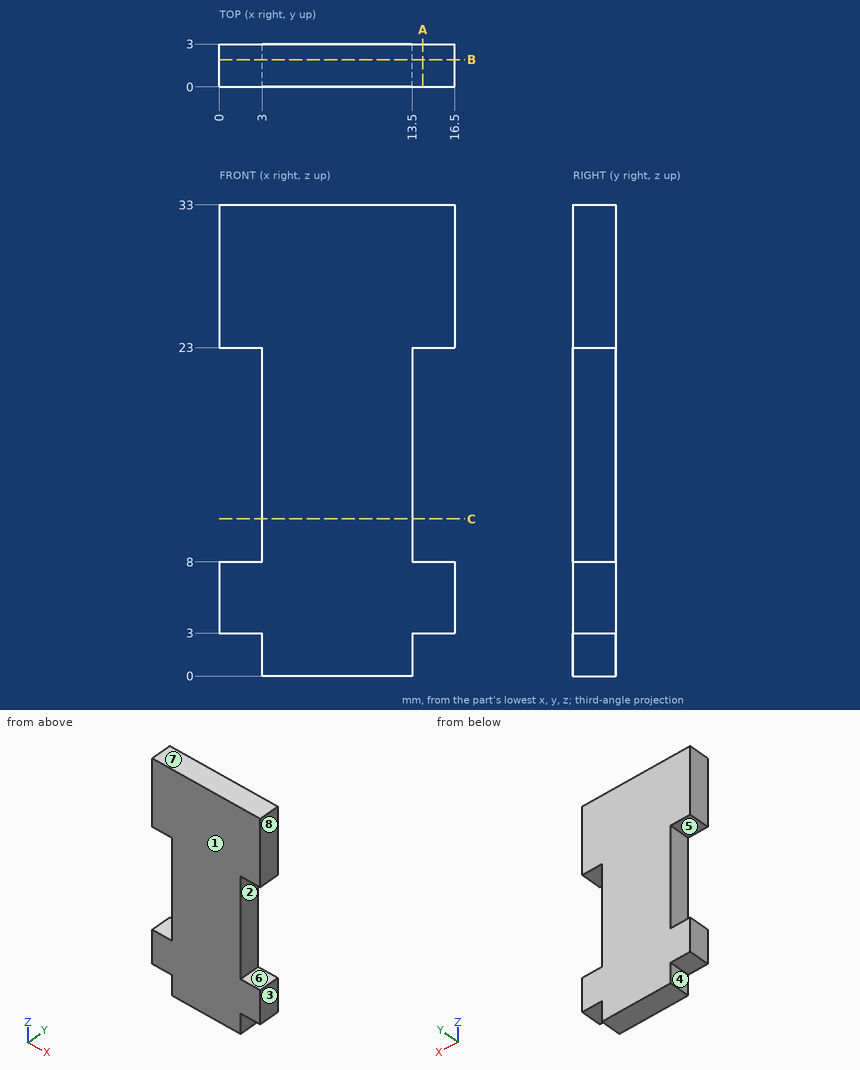
For this review, use the dimensioned drawing (mm, ordinates from the lowest corner) and the shaded views. A direction names the side the tool comes from. Give positions to 0.01 mm unless a question says otherwise; leave off trailing zeros. Write each loop counter-clockwise with the first axis right and the second up, starting at its lowest first coordinate (ties: lowest second). Pieces come first, ordered by that corner, then holes.
(1) Consider section C-C, the plane z = 11. Give the boundary of the cut face in (x, y), and give its area (3 significant figures).
(2) Tool access review of the marked faces 1, 2, 3, 4 and 5: name each direction out of +Z, -Z, +X, -X, +Y, -Y from which nothing blocks a thin tool from reaching the whole face with its end or side.
(3) Consider section A-A, the plane x = 14.25. Give the boundary of the cut face in (y, z).
(4) The part is to be moulded in two halves that separate along Z. For the marked faces 6, 7 and 8, say which applies: released by +Z, released by -Z, zero draft, split by the parting line, or undercut.
(5) For P1, Ø1.5, axis at x = 15.5, y = 2, coming from the -Z side; P2, Ø1.5, axis at y = 1.5, z = 12, coming from the +X side; P3, Ø0.9, axis at y = 1.5, z = 12, coming from the -X side, all flat-tipped, find the tip position at first contact; note any pin that passes through.
(6) Consider section B-B, the plane y = 1.9. Give the boundary of the cut face in (x, z).
(7) To check wall thickness, follow L1, parallel to Z at x = 1.5, y = 2.35; L2, parallel to X at y = 0.25, z = 18. State the ranges of each line that lie inside material, in increasing order.
Returned:
1. outline: (3, 0) - (13.5, 0) - (13.5, 3) - (3, 3) - close
1. area: 31.5 mm2
2. face 1: +Z, -Z, +X, -X, -Y
2. face 2: +X, +Y, -Y
2. face 3: +Z, -Z, +X, +Y, -Y
2. face 4: -Z, -X, +Y, -Y
2. face 5: -X, +Y, -Y
3. outline: (0, 3) - (3, 3) - (3, 8) - (0, 8) - close; (0, 23) - (3, 23) - (3, 33) - (0, 33) - close
4. face 6: undercut
4. face 7: released by +Z
4. face 8: zero draft
5. P1: stops at z = 3
5. P2: stops at x = 13.5
5. P3: stops at x = 3
6. outline: (0, 3) - (3, 3) - (3, 0) - (13.5, 0) - (13.5, 3) - (16.5, 3) - (16.5, 8) - (13.5, 8) - (13.5, 23) - (16.5, 23) - (16.5, 33) - (0, 33) - (0, 23) - (3, 23) - (3, 8) - (0, 8) - close
7. L1: z = 3 to 8, 23 to 33
7. L2: x = 3 to 13.5
